```python
from build123d import *

# Parameters (mm, degrees)
SCHIZZO1_R                   = 30
SCHIZZO1_R_2                 = 21
ESTRUSIONE_ESTRUSIONE1_DEPTH = 5
SCHIZZO7_R                   = 30
ESTRUSIONE_ESTRUSIONE2_DEPTH = 5
SCHIZZO3_R                   = 1.5
TAGLIO_ESTRUSIONE3_DEPTH     = 8
SCHIZZO10_R                  = 2.8
TAGLIO_ESTRUSIONE4_DEPTH     = 2.5
RIPETIZIONECIRCOLARE1_COUNT  = 6
SCHIZZO11_W                  = 14.5
SCHIZZO11_H                  = 17.5
ESTRUSIONE_ESTRUSIONE4_DEPTH = 29
SCHIZZO12_W                  = 20.5
SCHIZZO12_H                  = 20.5
TAGLIO_ESTRUSIONE5_DEPTH     = 31
RACCORDO3_R                  = 5
SCHIZZO13_R                  = 1.5
TAGLIO_ESTRUSIONE6_DEPTH     = 69.390423306
SCHIZZO14_R                  = 1.5
TAGLIO_ESTRUSIONE7_DEPTH     = 20
RACCORDO4_R                  = 4
RACCORDO5_R                  = 3
TAGLIO_ESTRUSIONE10_REACH    = 56.369
SCHIZZO15_R                  = 2.3
SCHIZZO16_R                  = 16.25
SCHIZZO16_R_2                = 2.3
TAGLIO_ESTRUSIONE11_DEPTH    = 2
SCHIZZO17_R                  = 4.35
TAGLIO_ESTRUSIONE12_DEPTH    = 3.5
SCHIZZO18_R                  = 4.35
TAGLIO_ESTRUSIONE13_DEPTH    = 20.5
SCHIZZO20_R                  = 2.5
TAGLIO_ESTRUSIONE14_DEPTH    = 50.117843051


with BuildPart() as part:
    # Schizzo1 → Estrusione-Estrusione1 (new body)
    with BuildSketch(Plane.XY):
        Circle(SCHIZZO1_R)
        Circle(SCHIZZO1_R_2, mode=Mode.SUBTRACT)
    extrude(amount=ESTRUSIONE_ESTRUSIONE1_DEPTH)

    # Schizzo7 → Estrusione-Estrusione2 (add)
    with BuildSketch(Plane.XY.offset(5)):
        Circle(SCHIZZO7_R)
    extrude(amount=ESTRUSIONE_ESTRUSIONE2_DEPTH)

    # Schizzo3 → Taglio-Estrusione3 (cut)
    with BuildSketch(Plane.XY):
        with Locations((0, 27.5)):
            Circle(SCHIZZO3_R)
    taglio_estrusione3 = extrude(amount=TAGLIO_ESTRUSIONE3_DEPTH, mode=Mode.SUBTRACT)

    # Schizzo10 → Taglio-Estrusione4 (cut)
    with BuildSketch(Plane.XY.offset(10)):
        with Locations((0, 27.5)):
            Circle(SCHIZZO10_R)
    taglio_estrusione4 = extrude(amount=-TAGLIO_ESTRUSIONE4_DEPTH, mode=Mode.SUBTRACT)

    # RipetizioneCircolare1: Taglio-Estrusione3, Taglio-Estrusione4 ×6 about axis
    ripetizionecircolare1_axis = Axis((0, 0, 0), (0, 0, 1))
    add([taglio_estrusione3.rotate(ripetizionecircolare1_axis, i * 360 / RIPETIZIONECIRCOLARE1_COUNT) for i in range(1, RIPETIZIONECIRCOLARE1_COUNT)], mode=Mode.SUBTRACT)
    add([taglio_estrusione4.rotate(ripetizionecircolare1_axis, i * 360 / RIPETIZIONECIRCOLARE1_COUNT) for i in range(1, RIPETIZIONECIRCOLARE1_COUNT)], mode=Mode.SUBTRACT)

    # Schizzo11 → Estrusione-Estrusione4 (add)
    with BuildSketch(Plane.XY.offset(10)):
        Polygon((-14.5, 17.5), (14.5, -17.5), (-14.5, -17.5), (-20.5, -17.5), (-20.5, 17.5), align=None)
        Polygon((0, 17.5), (-14.5, 17.5), (0, 0), align=None)
        with Locations((7.25, 8.75)):
            Rectangle(SCHIZZO11_W, SCHIZZO11_H)
        Polygon((14.5, 0), (0, 0), (14.5, -17.5), align=None)
    extrude(amount=ESTRUSIONE_ESTRUSIONE4_DEPTH)

    # Schizzo12 → Taglio-Estrusione5 (cut)
    with BuildSketch(Plane(origin=(14.5, 0, 0), x_dir=(0, 0, -1), z_dir=(1, 0, 0))):
        with Locations((-24.5, 0)):
            Rectangle(SCHIZZO12_W, SCHIZZO12_H)
    extrude(amount=-TAGLIO_ESTRUSIONE5_DEPTH, mode=Mode.SUBTRACT)

    # Raccordo3
    raccordo3_edges = [part.edges().sort_by_distance(p)[0] for p in [
        (-3, 17.5, 39),
        (-3, -17.5, 39),
    ]]
    fillet(raccordo3_edges, radius=RACCORDO3_R)

    # Schizzo13 → Taglio-Estrusione6 (cut, through all)
    with BuildSketch(Plane.XZ.offset(17.5)):
        with Locations(Location((0, 24.5, 0), (0, 0, 270))):
            Circle(SCHIZZO13_R)
    extrude(amount=-TAGLIO_ESTRUSIONE6_DEPTH, mode=Mode.SUBTRACT)

    # Schizzo14 → Taglio-Estrusione7 (cut)
    with BuildSketch(Plane.XY.offset(39)):
        Circle(SCHIZZO14_R)
    extrude(amount=-TAGLIO_ESTRUSIONE7_DEPTH, mode=Mode.SUBTRACT)

    # Raccordo4
    raccordo4_edges = [part.edges().sort_by_distance(p)[0] for p in [
        (14.5, 0, 10),
        (-3, -17.5, 10),
        (-3, 17.5, 10),
    ]]
    fillet(raccordo4_edges, radius=RACCORDO4_R)

    # Raccordo5
    raccordo5_edges = [part.edges().sort_by_distance(p)[0] for p in [
        (-20.5, -17.5, 24),
        (-20.5, 0, 39),
        (-20.5, 17.5, 24),
        (-20.5, 16.035533906, 37.535533906),
        (-20.5, -16.035533906, 37.535533906),
        (-20.5, 18.671572875, 11.171572875),
        (-20.5, -18.671572875, 11.171572875),
    ]]
    fillet(raccordo5_edges, radius=RACCORDO5_R)

    # Taglio-Estrusione10: up to this face of the body (flat: up to its plane)
    taglio_estrusione10_end = Plane(part.part.faces().sort_by_distance((-1, 0, 14.25))[0])
    # Schizzo15 → Taglio-Estrusione10 (cut, up to the picked face)
    with BuildSketch(Plane(origin=(0, 0, 5), x_dir=(-1, 0, 0), z_dir=(0, 0, -1)), mode=Mode.PRIVATE) as taglio_estrusione10_sk1:
        with Locations((13, 0)):
            Circle(SCHIZZO15_R)
    taglio_estrusione10_tool1 = split(extrude(taglio_estrusione10_sk1.sketch, amount=-TAGLIO_ESTRUSIONE10_REACH, mode=Mode.PRIVATE), bisect_by=taglio_estrusione10_end, keep=Keep.BOTH, mode=Mode.PRIVATE)
    # Schizzo15 → Taglio-Estrusione10 (cut, up to the picked face)
    with BuildSketch(Plane(origin=(0, 0, 5), x_dir=(-1, 0, 0), z_dir=(0, 0, -1)), mode=Mode.PRIVATE) as taglio_estrusione10_sk2:
        with Locations((-13, 0)):
            Circle(SCHIZZO15_R)
    taglio_estrusione10_tool2 = split(extrude(taglio_estrusione10_sk2.sketch, amount=-TAGLIO_ESTRUSIONE10_REACH, mode=Mode.PRIVATE), bisect_by=taglio_estrusione10_end, keep=Keep.BOTH, mode=Mode.PRIVATE)
    add(taglio_estrusione10_tool1.solids().sort_by(Axis((-13, 0, 5), (0, 0, 1)))[0], mode=Mode.SUBTRACT)
    add(taglio_estrusione10_tool2.solids().sort_by(Axis((13, 0, 5), (0, 0, 1)))[0], mode=Mode.SUBTRACT)

    # Schizzo16 → Taglio-Estrusione11 (cut)
    with BuildSketch(Plane(origin=(0, 0, 5), x_dir=(-1, 0, 0), z_dir=(0, 0, -1))):
        Circle(SCHIZZO16_R)
        with Locations((-13, 0)):
            Circle(SCHIZZO16_R_2, mode=Mode.SUBTRACT)
        with Locations((13, 0)):
            Circle(SCHIZZO16_R_2, mode=Mode.SUBTRACT)
    extrude(amount=-TAGLIO_ESTRUSIONE11_DEPTH, mode=Mode.SUBTRACT)

    # Schizzo17 → Taglio-Estrusione12 (cut)
    with BuildSketch(Plane.XY.offset(14.25)):
        with Locations((-13, 0)):
            Circle(SCHIZZO17_R)
        with Locations((13, 0)):
            Circle(SCHIZZO17_R)
    extrude(amount=-TAGLIO_ESTRUSIONE12_DEPTH, mode=Mode.SUBTRACT)

    # Schizzo18 → Taglio-Estrusione13 (cut)
    with BuildSketch(Plane.XY.offset(14.25)):
        with Locations((-13, 0)):
            Circle(SCHIZZO18_R)
        with Locations((13, 0)):
            Circle(SCHIZZO18_R)
    extrude(amount=TAGLIO_ESTRUSIONE13_DEPTH, mode=Mode.SUBTRACT)

    # Schizzo20 → Taglio-Estrusione14 (cut, through all)
    with BuildSketch(Plane.XY.offset(14.25)):
        with Locations((-13, 0)):
            Circle(SCHIZZO20_R)
        with BuildLine():
            Line((13, 2.5), (15.5, 2.5))
            Line((15.5, 2.5), (15.5, -2.5))
            Line((15.5, -2.5), (13, -2.5))
            ThreePointArc((13, -2.5), (10.5, 0), (13, 2.5))
        make_face()
    extrude(amount=TAGLIO_ESTRUSIONE14_DEPTH, mode=Mode.SUBTRACT)


solid = part.part
```
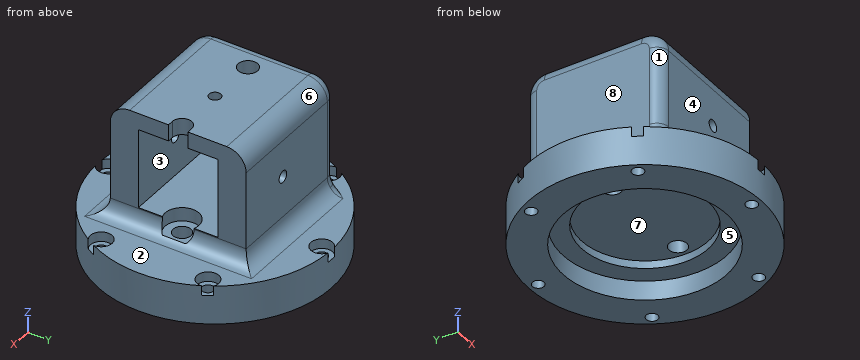
Verification items for the finished model (mm, model axes). Face numbers are marked on the shaded views. A direction names the side the tool comes from. Coordinates: 2 decimals unless noted, no trailing zeros. Loops run counter-clockwise (first coordinate to the right, second up) from the corner with the lowest first, then second, coordinate; pieces in that order, holes last. Notation, with made-up numbers: (47.25, 34) -> (64.25, 34) arc R29 ccw to (64.25, 60) -> close; hole circle Ø4 at (22, 55). An arc over 180 degrees is marked (long way). Answer in a Markdown table with one row per item. Add a question column.
1. Section check C-C, the plane z = 18. Enter the section's corners in (x, y), then the cut area to 3 significant figures.
2. Draft check along Y on the marked faces 6, 7 and 8. Enter one of: +Y half, -Y half, draft (parallel to the pull), parting line (faces both ways), or undercut.
3. Section check A-A, the plane z = 24.5. Enter the section's corners in (x, y).
4. Depth check by flat-ended pin: P1, Ø6, axis at x = -7, y = -1, coming from the -Z side; P2, Ø4, axis at x = 0, z = 24.5, coming from the +Y side; P3, Ø1, axis at x = 0.5, z = 34.5, coming from the -Y side; P4, Ø1.7, axis at x = -23.5, y = -14, coming from the +Z side. Enter the tip coordinate at first touch or a pass-through.
5. Section check B-B, the plane y = 27.5. Enter the section's corners in (x, z).
6. Material ranges on probe 1 along Y at (x, z) = (0, 6.55); probe 2 along X at (y, z) = (-13, 4); probe 3 along Z at (x, y) = (-17, -1), recorded low to high. Write a range as [from, to].
7. Section check D-D, the plane x = 0. Give the number of separate pieces and of enclosed holes in the cut face, then the cut area to 3 significant figures.
8. Access from +Z, -Z, +X, -X, +Y, -Y to the whole of each face (thin tool, end or side, straight path). Record for the marked faces 1, 2, 3, 4 and 5.
Derived:
| question | item | result |
|---|---|---|
| 1 | outline | (-20.5, -14.5) arc R3 ccw to (-17.5, -17.5) -> (14.5, -17.5) -> (14.5, -10.25) -> (-16.5, -10.25) -> (-16.5, -2.58) arc R4.35 cw to (-16.5, 2.58) -> (-16.5, 10.25) -> (14.5, 10.25) -> (14.5, 17.5) -> (-17.5, 17.5) arc R3 ccw to (-20.5, 14.5) -> close |
| 1 | area | 583 mm² |
| 2 | face 6 | +Y half |
| 2 | face 7 | undercut |
| 2 | face 8 | draft |
| 3 | outline | (-20.5, -14.5) arc R3 ccw to (-17.5, -17.5) -> (-1.5, -17.5) -> (-1.5, -10.25) -> (-16.5, -10.25) -> (-16.5, -2.58) arc R4.35 cw to (-16.5, 2.58) -> (-16.5, 10.25) -> (-1.5, 10.25) -> (-1.5, 17.5) -> (-17.5, 17.5) arc R3 ccw to (-20.5, 14.5) -> close; (1.5, -17.5) -> (14.5, -17.5) -> (14.5, -10.25) -> (1.5, -10.25) -> close; (1.5, 10.25) -> (14.5, 10.25) -> (14.5, 17.5) -> (1.5, 17.5) -> close |
| 4 | P1 | stops at z = 7 |
| 4 | P2 | stops at y = 17.5 |
| 4 | P3 | stops at y = -17.5 |
| 4 | P4 | passes through |
| 5 | outline | (-11.99, 0) -> (-1.5, 0) -> (-1.5, 7.5) -> (-2.8, 7.5) -> (-2.8, 10) -> (-11.99, 10) -> close; (1.5, 0) -> (11.99, 0) -> (11.99, 10) -> (2.8, 10) -> (2.8, 7.5) -> (1.5, 7.5) -> close |
| 6 | probe 1 | y = [-30, -29], [-26, -16.25], [16.25, 26], [29, 30] |
| 6 | probe 2 | x = [-27.04, -25.11], [-22.52, -16.49], [16.49, 22.52], [25.11, 27.04] |
| 6 | probe 3 | z = [5, 10.75], [34.75, 39] |
| 7 | separate pieces | 5 |
| 7 | enclosed holes | 0 |
| 7 | area | 788 mm² |
| 8 | face 1 | +Z, -X, -Y |
| 8 | face 2 | +Z |
| 8 | face 3 | +X |
| 8 | face 4 | +Z, +X, -X, -Y |
| 8 | face 5 | -Z |
